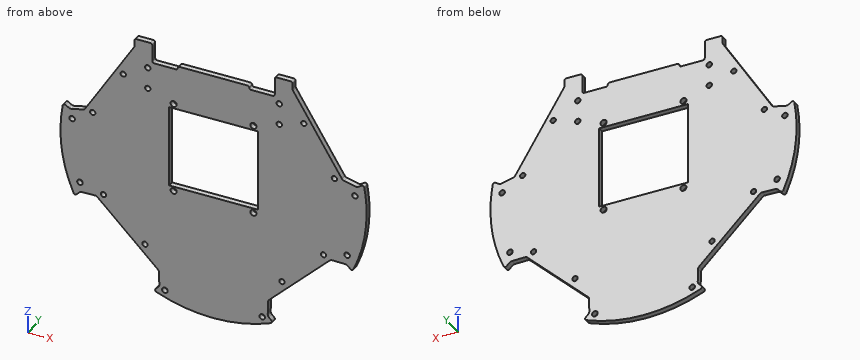
from build123d import *

# Parameters (mm, degrees)
BOSS_EXTRUDE4_DEPTH  = 1.5875
M3_CLEARANCE_HOLE3_D = 3
M3_CLEARANCE_HOLE1_D = 3.1
M3_CLEARANCE_HOLE4_D = 2.95
M3_CLEARANCE_HOLE2_D = 3.1
BOSS_EXTRUDE6_DEPTH  = 3.175
FILLET1_R            = 2
FILLET3_R            = 1
M3_CLEARANCE_HOLE5_D = 3.4
SKETCH27_W           = 49.3
SKETCH27_H           = 45.5
CUT_EXTRUDE5_DEPTH   = 10


with BuildPart() as part:
    # Sketch1 → Boss-Extrude4 (new, symmetric)
    with BuildSketch(Plane(origin=(0, 0, 0), x_dir=(1, 0, 0), z_dir=(0, 1, 0))):
        with BuildLine():
            Line((-62.799553621, 32.496136604), (-73.969425011, 32.691107434))
            Line((-73.969425011, 32.691107434), (-77.053684287, 35.88495141))
            ThreePointArc((-77.053684287, 35.88495141), (-84.36642289, 10.358894189), (-83.446216027, -16.178041625))
            Line((-83.446216027, -16.178041625), (-79.680911643, -13.825218315))
            Line((-79.680911643, -13.825218315), (-69.484649137, -16.179210996))
            Line((-69.484649137, -16.179210996), (-43.894490772, -57.132025032))
            Line((-43.894490772, -57.132025032), (-43.894490772, -64.826600275))
            Line((-43.894490772, -64.826600275), (-43.094490772, -64.826600275))
            Line((-43.094490772, -64.826600275), (-34, -64.826600275))
            Line((-34, -64.826600275), (-34, -55.55))
            Line((-34, -55.55), (-34, -53.55))
            Line((-34, -53.55), (-20, -53.55))
            Line((-20, -53.55), (-19.718918331, -55.55))
            Line((-19.718918331, -55.55), (19.718918331, -55.55))
            Line((19.718918331, -55.55), (20, -53.55))
            Line((20, -53.55), (34, -53.55))
            Line((34, -53.55), (34, -55.55))
            Line((34, -55.55), (34, -64.826600275))
            Line((34, -64.826600275), (43.094490772, -64.826600275))
            Line((43.094490772, -64.826600275), (43.894490772, -64.826600275))
            Line((43.894490772, -64.826600275), (43.894490772, -57.132025032))
            Line((43.894490772, -57.132025032), (69.484649137, -16.179210996))
            Line((69.484649137, -16.179210996), (79.680911643, -13.825218315))
            Line((79.680911643, -13.825218315), (83.446216027, -16.178041625))
            ThreePointArc((83.446216027, -16.178041625), (84.610662337, -8.126242604), (85, 0))
            ThreePointArc((85, 0), (82.98964744, 18.377116688), (77.053684287, 35.88495141))
            Line((77.053684287, 35.88495141), (73.969425011, 32.691107434))
            Line((73.969425011, 32.691107434), (62.799553621, 32.496136604))
            Line((62.799553621, 32.496136604), (30.284668021, 63.895396642))
            Line((30.284668021, 63.895396642), (30.089697191, 75.065268032))
            Line((30.089697191, 75.065268032), (33.173956467, 78.259112008))
            ThreePointArc((33.173956467, 78.259112008), (0, 85), (-33.173956467, 78.259112008))
            Line((-33.173956467, 78.259112008), (-30.089697191, 75.065268032))
            Line((-30.089697191, 75.065268032), (-30.284668021, 63.895396642))
            Line((-30.284668021, 63.895396642), (-62.799553621, 32.496136604))
        make_face()
    extrude(amount=BOSS_EXTRUDE4_DEPTH, both=True)

    # M3 Clearance Hole3 (through all)
    with Locations(Plane(origin=(0, -1.5875, 0), x_dir=(-1, 0, 0), z_dir=(0, -1, 0))):
        with Locations((36.5, -50), (36.5, -38), (-36.5, -50), (-36.5, -38)):
            Hole(M3_CLEARANCE_HOLE3_D / 2)

    # M3 Clearance Hole1 (through all)
    with Locations(Plane(origin=(0, 1.5875, 0), x_dir=(1, 0, 0), z_dir=(0, 1, 0))):
        with Locations((-78.542321426, -8.49139241), (78.542321426, -8.49139241), (74.155025063, 27.240269049), (-74.155025063, 27.240269049)):
            Hole(M3_CLEARANCE_HOLE1_D / 2)

    # M3 Clearance Hole4 (through all)
    with Locations(Plane(origin=(0, -1.5875, 0), x_dir=(-1, 0, 0), z_dir=(0, -1, 0))):
        with Locations((-67.099301622, -15.278865202), (-50.141885166, -42.416404279), (-61.062544382, 30.698137949), (-38.043670771, 52.927205804), (50.141885166, -42.416404279), (67.099301622, -15.278865202), (38.043670771, 52.927205804), (61.062544382, 30.698137949)):
            Hole(M3_CLEARANCE_HOLE4_D / 2)

    # M3 Clearance Hole2 (through all)
    with Locations(Plane(origin=(0, 1.5875, 0), x_dir=(1, 0, 0), z_dir=(0, 1, 0))):
        with Locations((27, 76.497766718), (-27, 76.497766718)):
            Hole(M3_CLEARANCE_HOLE2_D / 2)

    # Sketch22 → Boss-Extrude6 (add)
    with BuildSketch(Plane(origin=(0, 1.5875, 0), x_dir=(1, 0, 0), z_dir=(0, 1, 0))):
        Polygon((65.061950694, 32.535626892), (30.245177733, 66.157793715), (30.284668021, 63.895396642), (62.799553621, 32.496136604), align=None)
        Polygon((-30.284668021, 63.895396642), (-30.245177733, 66.157793715), (-65.061950694, 32.535626892), (-62.799553621, 32.496136604), align=None)
        Polygon((43.894490772, -60.151352895), (71.689396914, -15.670204865), (69.484649137, -16.179210996), (43.894490772, -57.132025032), align=None)
        Polygon((-69.484649137, -16.179210996), (-71.689396914, -15.670204865), (-43.894490772, -60.151352895), (-43.894490772, -57.132025032), align=None)
    extrude(amount=-BOSS_EXTRUDE6_DEPTH)

    # Fillet1
    fillet1_edges = [part.edges().sort_by_distance(p)[0] for p in [
        (-30.245177733, -0.79375, -66.157793715),
        (-65.061950694, -0.79375, -32.535626892),
        (-71.689396914, -0.79375, 15.670204865),
        (-43.894490772, -0.79375, 60.151352895),
        (43.894490772, 0.79375, 60.151352895),
        (71.689396914, 0.79375, 15.670204865),
        (65.061950694, -0.79375, -32.535626892),
        (30.245177733, 0.79375, -66.157793715),
        (30.089697191, -0.79375, -75.065268032),
        (73.969425011, -0.79375, -32.691107434),
        (79.680911643, -0.79375, 13.825218315),
        (-79.680911643, -0.79375, 13.825218315),
        (-73.969425011, -0.79375, -32.691107434),
        (-30.089697191, -0.79375, -75.065268032),
    ]]
    fillet(fillet1_edges, radius=FILLET1_R)

    # Fillet3
    fillet3_edges = [part.edges().sort_by_distance(p)[0] for p in [
        (33.173956467, -0.79375, -78.259112008),
        (77.053684287, 0.79375, -35.88495141),
        (83.446216027, -0.79375, 16.178041625),
        (43.894490772, -0.79375, 64.826600275),
        (34, 0.79375, 64.826600275),
        (34, -0.79375, 53.55),
        (20, -0.79375, 53.55),
        (19.718918331, 0.79375, 55.55),
        (-19.718918331, 0.79375, 55.55),
        (-20, -0.79375, 53.55),
        (-34, -0.79375, 53.55),
        (-34, 0.79375, 64.826600275),
        (-43.894490772, -0.79375, 64.826600275),
        (-83.446216027, -0.79375, 16.178041625),
        (-77.053684287, -0.79375, -35.88495141),
        (-33.173956467, -0.79375, -78.259112008),
    ]]
    fillet(fillet3_edges, radius=FILLET3_R)

    # M3 Clearance Hole5 (through all)
    with Locations(Plane(origin=(0, 1.5875, 0), x_dir=(1, 0, 0), z_dir=(0, 1, 0))):
        with Locations((-22.15, 17.45), (-22.15, -33.05), (22.15, -33.05), (22.15, 17.45)):
            Hole(M3_CLEARANCE_HOLE5_D / 2)

    # Sketch27 → Cut-Extrude5 (cut)
    with BuildSketch(Plane(origin=(0, 1.5875, 0), x_dir=(1, 0, 0), z_dir=(0, 1, 0))):
        with Locations((0, -7.8)):
            Rectangle(SKETCH27_W, SKETCH27_H)
    extrude(amount=-CUT_EXTRUDE5_DEPTH, mode=Mode.SUBTRACT)


solid = part.part
Model file for the job. Use its own axes, mm. Coordinates: 2 decimals unless noted, no trailing zeros. Loops run counter-clockwise (first coordinate to the right, second up) from the corner with the lowest first, then second, coordinate; pieces in that order, holes last. Notation, with made-up numbers: (-36.5, -29.75) -> (-1.5, -29.75) arc R28 ccw to (-1.5, -3.75) -> close; hole circle Ø10 at (-28, 14.25). An arc over 180 degrees is marked (long way). Use one line per item in the form item = value. Start each with the question number.
(1) Flat gauge pins, fed straight in: pin 1 (1.5 mm diameter, centred on y = 0, z = -57, fed in from -X) (3 decimals); pin 2 (1.6 mm diameter, centred on x = -4, y = -0.5, fed in from -Z); pin 3 (1.5 mm diameter, centred on y = -1, z = -64, fed in from -X). Where does each tip first touch, or does it go through?
(2) Cut at A-A on x = 4.5. Give the cut face in (y, z).
(3) Cut at D-D on y = 0.75. Give the number of separate pieces and of enclosed holes in the cut face, and give its area (3 significant figures).
(4) Cut at C-C on z = -21. Give the cut face in (x, y), and give its area (3 significant figures).
(5) Cut at B-B on z = 21. Give the cut face in (x, y).
(6) Probe probe 1 along X at (y, z) = (0.5, 2); probe 2 along X at (y, z) = (0.9, 32); probe 3 along X at (y, z) = (-1.05, 9). List the from-to ranges inside material, lowest first. Write a range as from..to.
Values:
q1.pin_1 = -40.505
q1.pin_2 = -84.94
q1.pin_3 = -33.26
q2.outline = (-1.59, -84.88) -> (1.59, -84.88) -> (1.59, -14.95) -> (-1.59, -14.95) -> close; (-1.59, 30.55) -> (1.59, 30.55) -> (1.59, 55.55) -> (-1.59, 55.55) -> close
q3.separate_pieces = 1
q3.enclosed_holes = 23
q3.area = 14,700 mm2
q4.outline = (-82.37, -1.59) -> (82.37, -1.59) -> (82.37, 1.59) -> (-82.37, 1.59) -> close
q4.area = 523 mm2
q5.outline = (-68.36, -1.59) -> (-24.65, -1.59) -> (-24.65, 1.59) -> (-68.36, 1.59) -> close; (24.65, -1.59) -> (68.36, -1.59) -> (68.36, 1.59) -> (24.65, 1.59) -> close
q6.probe_1 = -84.98..-24.65, 24.65..84.98
q6.probe_2 = -61.49..-23.49, -20.81..20.81, 23.49..61.49
q6.probe_3 = -84.52..-80.01, -77.08..-24.65, 24.65..77.08, 80.01..84.52
